```python
from build123d import *

# Parameters (mm, degrees)
SKETCH1_W           = 90
SKETCH1_H           = 3
BOSS_EXTRUDE1_DEPTH = 30
SKETCH2_R           = 1.5
CUT_EXTRUDE1_DEPTH  = 20
CUT_EXTRUDE2_START  = 20
SKETCH2_3_R         = 3
SKETCH2_3_R_2       = 1.5
CUT_EXTRUDE2_DEPTH  = 20
CHAMFER1_SIZE       = 5


with BuildPart() as part:
    # Sketch1 → Boss-Extrude1 (new body)
    with BuildSketch(Plane(origin=(0, 0, 0), x_dir=(1, 0, 0), z_dir=(0, 1, 0))):
        with Locations((35, -4.607181)):
            Rectangle(SKETCH1_W, SKETCH1_H)
        Polygon((-5, -3.107181), (2, -3.107181), (2, 6.892819), (0, 6.892819), (0, 8.892819), (2, 8.892819), (2, 11.892819), (-3, 11.892819), align=None)
        Polygon((68, 6.892819), (68, -3.107181), (75, -3.107181), (73, 11.892819), (68, 11.892819), (68, 8.892819), (70, 8.892819), (70, 6.892819), align=None)
    extrude(amount=BOSS_EXTRUDE1_DEPTH)

    # Sketch2 → Cut-Extrude1 (cut)
    with BuildSketch(Plane(origin=(0, 0, 3.107181), x_dir=(-1, 0, 0), z_dir=(0, 0, -1))):
        with Locations((7, 7.154704)):
            Circle(SKETCH2_R)
        with Locations((-77, 7.154704)):
            Circle(SKETCH2_R)
    extrude(amount=-CUT_EXTRUDE1_DEPTH, mode=Mode.SUBTRACT)

    # Sketch2_3 → Cut-Extrude2 (cut)
    # profile 1 of 2: a face of its own
    with BuildSketch(Plane(origin=(0, 0, 3.107181), x_dir=(-1, 0, 0), z_dir=(0, 0, -1)).offset(CUT_EXTRUDE2_START)):
        with Locations((7, 7.154704)):
            Circle(SKETCH2_3_R)
        with Locations((7, 7.154704)):
            Circle(SKETCH2_3_R_2, mode=Mode.SUBTRACT)
    # profile 2 of 2: a face of its own
    with BuildSketch(Plane(origin=(0, 0, 3.107181), x_dir=(-1, 0, 0), z_dir=(0, 0, -1)).offset(CUT_EXTRUDE2_START)):
        with Locations((-77, 7.154704)):
            Circle(SKETCH2_3_R)
        with Locations((-77, 7.154704)):
            Circle(SKETCH2_3_R_2, mode=Mode.SUBTRACT)
    extrude(amount=-CUT_EXTRUDE2_DEPTH, mode=Mode.SUBTRACT)

    # Chamfer1
    chamfer1_edges = [part.edges().sort_by_distance(p)[0] for p in [
        (80, 0, 4.607181),
        (80, 30, 4.607181),
        (-10, 0, 4.607181),
        (-10, 30, 4.607181),
    ]]
    chamfer(chamfer1_edges, length=CHAMFER1_SIZE)


solid = part.part
```
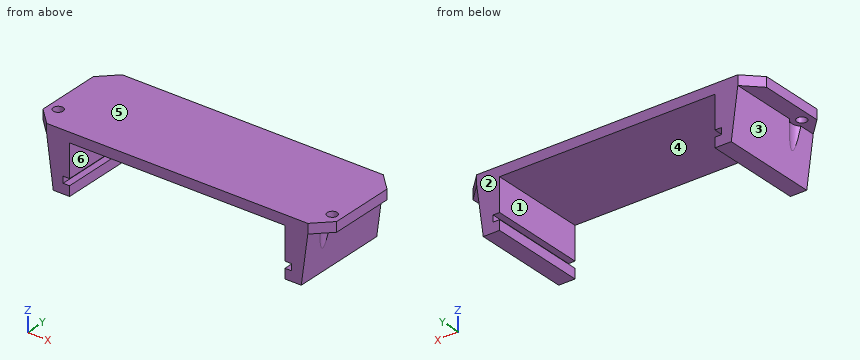
Work out the finished part from the listing and answer in its coordinate system (mm). Face numbers are marked on the shaded views. A direction names the side the tool comes from. Give positions to 0.01 mm unless a question says otherwise; leave off trailing zeros. Loops run counter-clockwise (first coordinate to the right, second up) from the corner with the lowest first, then second, coordinate; pieces in that order, holes last. Notation, with made-up numbers: (30, 34) - (47, 34) arc R17 cw to (47, 44) - close; hole circle Ø8 at (-2, 70). An arc over 180 degrees is marked (long way). One line per question, with ' | ' between items.
(1) The part is cut by section B-B (y = 23.5). Write down the section's boundary in (x, z).
Recorded:
outline: (-10, 3.11) - (-5, 3.11) - (-3, -11.89) - (2, -11.89) - (2, -8.89) - (0, -8.89) - (0, -6.89) - (2, -6.89) - (2, 3.11) - (68, 3.11) - (68, -6.89) - (70, -6.89) - (70, -8.89) - (68, -8.89) - (68, -11.89) - (73, -11.89) - (75, 3.11) - (80, 3.11) - (80, 6.11) - (-10, 6.11) - close
(2) The mould has two halves that part along X. Classify the marked faces 3, 4, 5 and 6: +X half, -X half, draft (parallel to the pull), parting line (faces both ways), or undercut.
Recorded:
face 3: -X half | face 4: undercut | face 5: draft | face 6: undercut
(3) Each of these flat-tipped pins is pushed along its axis until it touches: pin 1 Ø1 at (x, y) = (43, 20) entering from -Z; pin 2 Ø0.9 at (y, z) = (19.5, -11) entering from -X; pin 3 Ø1.6 at (y, z) = (11, -8) entering from -X. Where does it stop, or does it pass through?
Recorded:
pin 1: stops at z = 3.11 | pin 2: stops at x = -3.18 | pin 3: stops at x = -3.63
(4) Straight lines are drawn through the part: probe 1 along Z at (x, y) = (0.5, 23.5); probe 2 along X at (y, z) = (7.5, -0.25); probe 3 along Z at (x, y) = (57.5, 24.75). For each, find the intervals that lie inside material, in ascending order.
Recorded:
probe 1: z = -11.89 to -8.89, -6.89 to 6.11 | probe 2: x = -4.02 to 2, 68 to 74.02 | probe 3: z = 3.11 to 6.11
(5) The part is cut by section A-A (x = 77). Write down the section's boundary in (y, z), then the cut area to 3 significant figures.
Recorded:
outline: (2, 3.11) - (5.65, 3.11) - (5.65, 6.11) - (2, 6.11) - close; (8.65, 3.11) - (28, 3.11) - (28, 6.11) - (8.65, 6.11) - close | area: 69.0 mm²
(6) A tool of negligible diameter and unlimited length cuts with its end or side. For the marked faces 1 and 2, from which of +Z, -Z, +X, -X, +Y, -Y can it reach the whole face along a straight path? Write none if from no direction.
Recorded:
face 1: -Z, +Y, -Y | face 2: +Z, -Z, +X, -X, +Y
(7) The part is cut by section C-C (y = 3.75). Write down the section's boundary in (x, z), then the cut area to 4 significant figures.
Recorded:
outline: (-8.75, 3.11) - (-5, 3.11) - (-3, -11.89) - (2, -11.89) - (2, -8.89) - (0, -8.89) - (0, -6.89) - (2, -6.89) - (2, 3.11) - (68, 3.11) - (68, -6.89) - (70, -6.89) - (70, -8.89) - (68, -8.89) - (68, -11.89) - (73, -11.89) - (75, 3.11) - (78.75, 3.11) - (78.75, 6.11) - (-8.75, 6.11) - close | area: 434.5 mm²
